Could you check a few things on this model? Use its own coordinates, in mm. Face numbers are marked on the shaded views. A direction names the side the tool comes from. Give positions to 0.01 mm unless a question says otherwise; leave off trailing zeros. Write each loop counter-clockwise with the first axis right and the second up, starting at its lowest first coordinate (ties: lowest second). Pieces come first, ordered by that corner, then holes. Notation, with made-up numbers: (57, 51.25) - (81, 51.25) arc R4 cw to (81, 58.25) - close; hole circle Ø11 at (-24.75, 10.5). An arc over 180 degrees is marked (long way). Answer in a Markdown table with one row per item.
from build123d import *

# Parameters (mm, degrees)
SKETCH1_W           = 24
SKETCH1_H           = 24
BOSS_EXTRUDE2_DEPTH = 4
SKETCH3_R           = 6
BOSS_EXTRUDE3_DEPTH = 96


with BuildPart() as part:
    # Sketch1 → Boss-Extrude2 (new, symmetric)
    with BuildSketch(Plane.XY):
        Rectangle(SKETCH1_W, SKETCH1_H)
    extrude(amount=BOSS_EXTRUDE2_DEPTH, both=True)

    # Sketch3 → Boss-Extrude3 (add)
    with BuildSketch(Plane.XY.offset(4)):
        Circle(SKETCH3_R)
    extrude(amount=BOSS_EXTRUDE3_DEPTH)

    # Sketch5 → Cut-Revolve8 (revolve, cut)
    with BuildSketch(Plane(origin=(0, 0, 0), x_dir=(1, 0, 0), z_dir=(0, 1, 0)), mode=Mode.PRIVATE) as cut_revolve8_sk:
        with BuildLine():
            Line((0, 4), (6.30628562, 4))
            ThreePointArc((6.30628562, 4), (11.96313987, 1.656854249), (14.30628562, -4))
            Line((14.30628562, -4), (24.30628562, -4))
            ThreePointArc((24.30628562, -4), (15.122793398, 9.010065299), (0, 14))
            Line((0, 14), (0, 4))
        make_face()
    revolve(cut_revolve8_sk.sketch.rotate(Axis((0, 0, -4), (0, 0, 1)), 180), axis=Axis((0, 0, -4), (0, 0, 1)), mode=Mode.SUBTRACT)


solid = part.part
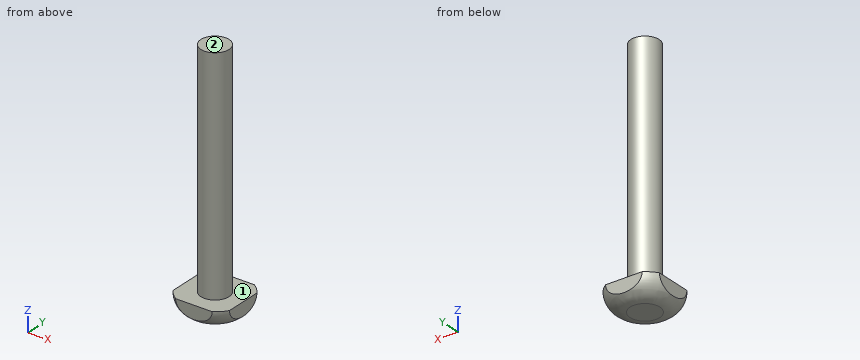
1) Will these pins go through, and if not, where does the flat tip stop? P1, Ø6, axis at x = -9.5, y = -5.5, coming from the +Z side; P2, Ø12, axis at y = 2, z = 25.5, coming from the -X side; P3, Ø6, axis at x = -8.5, y = -6, coming from the -Z side.
Check values:
| item | result |
|---|---|
| P1 | stops at z = 4 |
| P2 | stops at x = -6 |
| P3 | stops at z = -3.92 |
2) On a 3-axis mill with a long thin cutter (end or side, diameter ignored), from which of +Z, -Z, +X, -X, +Y, -Y can I reach the whole of each face in a straight line? I mean the marked faces 1 and 2. Say none if no direction works.
Check values:
| item | result |
|---|---|
| face 1 | +Z |
| face 2 | +Z, +X, -X, +Y, -Y |
3) Imagine slicing it at A-A (z = 32). List the corners of the cut face in (x, y) for me, then the cut area to 3 significant figures.
Check values:
| item | result |
|---|---|
| outline | circle Ø12 at (0, 0) |
| area | 113 mm2 |
4) If I drill on line 1 (Y direction, x = 0.5, z = 33); line 2 (X direction, y = 2.5, z = 31.5); line 3 (Z direction, x = 7.25, y = 10.5), over which ranges is the centre line in solid material (lowest first)?
Check values:
| item | result |
|---|---|
| line 1 | y = -5.98 to 5.98 |
| line 2 | x = -5.45 to 5.45 |
| line 3 | z = -0.73 to 4 |
